CAD build for the part. Positions are in the model's coordinates, mm. A direction names the side the tool comes from. Give positions to 0.01 mm unless a question says otherwise; leave off trailing zeros. Loops run counter-clockwise (first coordinate to the right, second up) from the corner with the lowest first, then second, coordinate; pieces in that order, holes last. Notation, with made-up numbers: (58.5, 59) - (109.5, 59) arc R22 ccw to (109.5, 96) - close; hole circle Ø5 at (22, 4.25). An arc over 180 degrees is marked (long way). Return JSON: item names as keys, results as strings.
from build123d import *

# Parameters (mm, degrees)
BOSS_EXTRUDE1_DEPTH = 10
FILLET1_R           = 2
FILLET3_R           = 0.5
FILLET4_R           = 10
SKETCH2_R           = 1.875
CUT_EXTRUDE1_DEPTH  = 25.417106227
CUT_EXTRUDE2_START  = 6
SKETCH3_R           = 3
CUT_EXTRUDE2_DEPTH  = 10


with BuildPart() as part:
    # Sketch1 → Boss-Extrude1 (new body)
    with BuildSketch(Plane.XY):
        with BuildLine():
            Line((-18.986115361, 1), (-6.5743821, 1))
            ThreePointArc((-6.5743821, 1), (0, 6.65), (6.5743821, 1))
            Line((6.5743821, 1), (18.986115361, 1))
            Line((18.986115361, 1), (18.986115361, 6))
            Line((18.986115361, 6), (9.986115361, 6))
            ThreePointArc((9.986115361, 6), (0, 11.65), (-9.986115361, 6))
            Line((-9.986115361, 6), (-18.986115361, 6))
            Line((-18.986115361, 6), (-18.986115361, 1))
        make_face()
    extrude(amount=BOSS_EXTRUDE1_DEPTH)

    # Fillet1
    fillet1_edges = [part.edges().sort_by_distance(p)[0] for p in [
        (-18.986115361, 3.5, 0),
        (18.986115361, 3.5, 10),
        (-18.986115361, 3.5, 10),
        (18.986115361, 3.5, 0),
    ]]
    fillet(fillet1_edges, radius=FILLET1_R)

    # Fillet3
    fillet3_edges = [part.edges().sort_by_distance(p)[0] for p in [
        (6.5743821, 1, 5),
        (-6.5743821, 1, 5),
    ]]
    fillet(fillet3_edges, radius=FILLET3_R)

    # Fillet4
    fillet4_edges = [part.edges().sort_by_distance(p)[0] for p in [
        (-9.986115361, 6, 5),
        (9.986115361, 6, 5),
    ]]
    fillet(fillet4_edges, radius=FILLET4_R)

    # Sketch2 → Cut-Extrude1 (cut, through all)
    with BuildSketch(Plane(origin=(0, 0, 0), x_dir=(1, 0, 0), z_dir=(0, 1, 0))):
        with Locations(Location((-15.1, -5, 0), (0, 0, 74.058148942))):
            Circle(SKETCH2_R)
        with Locations(Location((15.1, -5, 0), (0, 0, 105.941851061))):
            Circle(SKETCH2_R)
    extrude(amount=CUT_EXTRUDE1_DEPTH, mode=Mode.SUBTRACT)

    # Sketch3 → Cut-Extrude2 (cut)
    with BuildSketch(Plane(origin=(0, 0, 0), x_dir=(1, 0, 0), z_dir=(0, 1, 0)).offset(CUT_EXTRUDE2_START)):
        with Locations((-15.1, -5)):
            Circle(SKETCH3_R)
        with Locations((15.1, -5)):
            Circle(SKETCH3_R)
    extrude(amount=CUT_EXTRUDE2_DEPTH, mode=Mode.SUBTRACT)


solid = part.part
1. Drop flat-ended pins along their axis: P1, Ø4, axis at x = 11.5, z = 8.5, coming from the +Y side; P2, Ø4, axis at x = -8.5, z = 2.5, coming from the +Y side; P3, Ø3, axis at x = -8.5, z = 6.5, coming from the +Y side. Give the stop position or say it passes through.
Values follow:
{"P1": "stops at y = 7.39", "P2": "stops at y = 9.67", "P3": "stops at y = 9.31"}
2. Cut at B-B, the plane z = 5. Write the cut outline in (x, y) (3 decimals).
Values follow:
{"outline": "(-18.986, 1) - (-16.975, 1) - (-16.975, 6) - (-18.986, 6) - close; (-13.225, 1) - (-6.991, 1) arc R0.5 ccw to (-6.502, 1.395) arc R6.65 cw to (6.502, 1.395) arc R0.5 ccw to (6.991, 1) - (13.225, 1) - (13.225, 6) - (12.1, 6) - (12.1, 6.314) arc R10 cw to (7.848, 8.61) arc R11.65 ccw to (-7.848, 8.61) arc R10 cw to (-12.1, 6.314) - (-12.1, 6) - (-13.225, 6) - close; (16.975, 1) - (18.986, 1) - (18.986, 6) - (16.975, 6) - close"}
3. Cut at A-A, the plane x = 15.1. Write the cut outline in (y, z) (3 decimals), plus the area to 4 significant figures.
Values follow:
{"outline": "(1, 0) - (6, 0) - (6, 3.125) - (1, 3.125) - close; (1, 6.875) - (6, 6.875) - (6, 10) - (1, 10) - close", "area": "31.25 mm²"}
4. Drill centre lines: probe 1 along Z at (x, y) = (15.1, 3.6) (3 decimals); probe 2 along X at (y, z) = (3, 5) (3 decimals); probe 3 along X at (y, z) = (4, 4). Where is each one in solid material? Low to high.
Values follow:
{"probe 1": "z = 0 to 3.125, 6.875 to 10", "probe 2": "x = -18.986 to -16.975, -13.225 to -5.935, 5.935 to 13.225, 16.975 to 18.986", "probe 3": "x = -18.99 to -16.69, -13.51 to -5.31, 5.31 to 13.51, 16.69 to 18.99"}
5. Cut at C-C, the plane y = 4.5. Write the cut outline in (x, z) (3 decimals), plus the area to 3 significant figures.
Values follow:
{"outline": "(-18.986, 2) arc R2 ccw to (-16.986, 0) - (-4.896, 0) - (-4.896, 10) - (-16.986, 10) arc R2 ccw to (-18.986, 8) - close; (4.896, 0) - (16.986, 0) arc R2 ccw to (18.986, 2) - (18.986, 8) arc R2 ccw to (16.986, 10) - (4.896, 10) - close; hole circle Ø3.75 at (-15.1, 5); hole circle Ø3.75 at (15.1, 5)", "area": "256 mm²"}
6. Pull direction Y, two halves, no side cores. Call faces 4 (the face through (-13, 1, 5)), 5 (the face through (-15.15, 3.465, 3.126)), 6 (the face through (-10.27, 6.98, 5.07)): +Y half, -Y half, draft (parallel to the pull), parting line (faces both ways), or undercut.
Values follow:
{"face 4": "-Y half", "face 5": "draft", "face 6": "+Y half"}
7. Which spindle directions (+Z, -Z, +X, -X, +Y, -Y) get a long thin tool onto all of the face, cutting with end or side? Do faces 1 (the face through (0.12, 11.65, 4.93)), 2 (the face through (-17, 6, 6)), 3 (the face through (17, 6, 6)). Say none if no direction does.
Values follow:
{"face 1": "+Z, -Z, +Y", "face 2": "-X, +Y", "face 3": "+X, +Y"}
8. Cut at D-D, the plane z = 8.5. Write the cut outline in (x, y) (3 decimals), plus the area to 3 significant figures.
Values follow:
{"outline": "(-18.923, 1) - (-6.991, 1) arc R0.5 ccw to (-6.502, 1.395) arc R6.65 cw to (6.502, 1.395) arc R0.5 ccw to (6.991, 1) - (18.923, 1) - (18.923, 6) - (14.585, 6) arc R10 cw to (7.848, 8.61) arc R11.65 ccw to (-7.848, 8.61) arc R10 cw to (-14.585, 6) - (-18.923, 6) - close", "area": "218 mm²"}
